Build history of the part. All positions in model axes, mm. Round coordinates to 2 decimals unless told otherwise and drop trailing zeros. Write each loop counter-clockwise with the first axis right and the second up, starting at its lowest first coordinate (ties: lowest second). Pieces come first, ordered by that corner, then holes. Notation, with made-up numbers: (-23, 59) -> (-8, 59) arc R9 cw to (-8, 69) -> close; hole circle Ø10 at (7, -2.75). An arc over 180 degrees is marked (long way). Return JSON: item names as keys, results as strings.
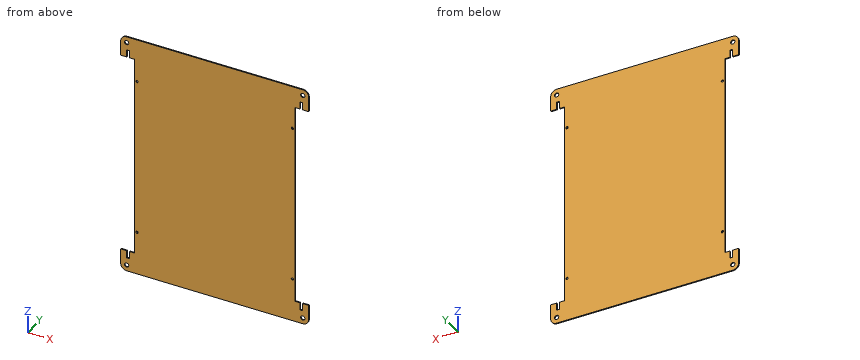
from build123d import *

# Parameters (mm, degrees)
SKETCH1_W                  = 254
SKETCH1_H                  = 326
BOSS_EXTRUDE1_DEPTH        = 1.51892
M2_5_CLEARANCE_HOLE1_D     = 3.1
M2_5_CLEARANCE_HOLE1_DEPTH = 11.938
M2_5_CLEARANCE_HOLE1_TIP   = 0.931333959
M5_CLEARANCE_HOLE1_D       = 5.8
M5_CLEARANCE_HOLE1_DEPTH   = 11.938
M5_CLEARANCE_HOLE1_TIP     = 1.742495795
FILLET1_R                  = 8
SKETCH6_W                  = 4
SKETCH6_H                  = 10
CUT_EXTRUDE1_DEPTH         = 10


with BuildPart() as part:
    # Sketch1 → Boss-Extrude1 (new body)
    with BuildSketch(Plane(origin=(0, 0, 0), x_dir=(1, 0, 0), z_dir=(0, 1, 0))):
        Rectangle(SKETCH1_W, SKETCH1_H)
    extrude(amount=BOSS_EXTRUDE1_DEPTH)

    # M2.5 Clearance Hole1
    with Locations(Plane(origin=(-105, 1.51892, 105), x_dir=(0, 0, 1), z_dir=(0, 1, 0))):
        with Locations((0, 0), (-210, 0), (-210, 210), (0, 210)):
            Hole(M2_5_CLEARANCE_HOLE1_D / 2, depth=M2_5_CLEARANCE_HOLE1_DEPTH)
            with Locations((0, 0, -(M2_5_CLEARANCE_HOLE1_DEPTH + M2_5_CLEARANCE_HOLE1_TIP / 2))):  # 118° drill point
                Cone(0, M2_5_CLEARANCE_HOLE1_D / 2, M2_5_CLEARANCE_HOLE1_TIP, mode=Mode.SUBTRACT)

    # M5 Clearance Hole1
    with Locations(Plane(origin=(0, 1.51892, 0), x_dir=(1, 0, 0), z_dir=(0, 1, 0))):
        with Locations((-119, 155), (119, 155), (119, -155), (-119, -155)):
            Hole(M5_CLEARANCE_HOLE1_D / 2, depth=M5_CLEARANCE_HOLE1_DEPTH)
            with Locations((0, 0, -(M5_CLEARANCE_HOLE1_DEPTH + M5_CLEARANCE_HOLE1_TIP / 2))):  # 118° drill point
                Cone(0, M5_CLEARANCE_HOLE1_D / 2, M5_CLEARANCE_HOLE1_TIP, mode=Mode.SUBTRACT)

    # Fillet1
    fillet1_edges = [part.edges().sort_by_distance(p)[0] for p in [
        (-127, 0.75946, -163),
        (127, 0.75946, -163),
        (127, 0.75946, 163),
        (-127, 0.75946, 163),
    ]]
    fillet(fillet1_edges, radius=FILLET1_R)

    # Sketch6 → Cut-Extrude1 (cut)
    with BuildSketch(Plane(origin=(0, 1.51892, 0), x_dir=(1, 0, 0), z_dir=(0, 1, 0))):
        Polygon((127, -135), (127, 135), (119, 135), (115, 135), (108.5, 135), (108.5, -135), (115, -135), (119, -135), align=None)
        with Locations((117, -140)):
            Rectangle(SKETCH6_W, SKETCH6_H)
        with Locations((117, 140)):
            Rectangle(SKETCH6_W, SKETCH6_H)
        Polygon((-119, -135), (-115, -135), (-108.5, -135), (-108.5, 135), (-115, 135), (-119, 135), (-127, 135), (-127, -135), align=None)
        with Locations((-117, -140)):
            Rectangle(SKETCH6_W, SKETCH6_H)
        with Locations((-117, 140)):
            Rectangle(SKETCH6_W, SKETCH6_H)
    extrude(amount=-CUT_EXTRUDE1_DEPTH, mode=Mode.SUBTRACT)


solid = part.part
Q1. Wall check: L1, parallel to Z at x = 105, y = 1; L2, parallel to X at y = 0.6, z = -141; L3, parallel to X at y = 0.6, z = -155. Give the ranges that are in metal, low to high.
Verdict:
{"L1": "z = -163 to -106.55, -103.45 to 103.45, 106.55 to 163", "L2": "x = -127 to -119, -115 to 115, 119 to 127", "L3": "x = -127 to -121.9, -116.1 to 116.1, 121.9 to 127"}
Q2. Saw through at B-B on y = 0.6. Count the separate pieces of the cut face and the enclosed holes in it, then the cut area to 3 significant figures.
Verdict:
{"separate pieces": "1", "enclosed holes": "8", "area": "72,500 mm²"}
Q3. Saw through at A-A on z = -8.5. List the corners of the cut face in (x, y), then the cut area to 3 significant figures.
Verdict:
{"outline": "(-108.5, 0) -> (108.5, 0) -> (108.5, 1.52) -> (-108.5, 1.52) -> close", "area": "330 mm²"}
